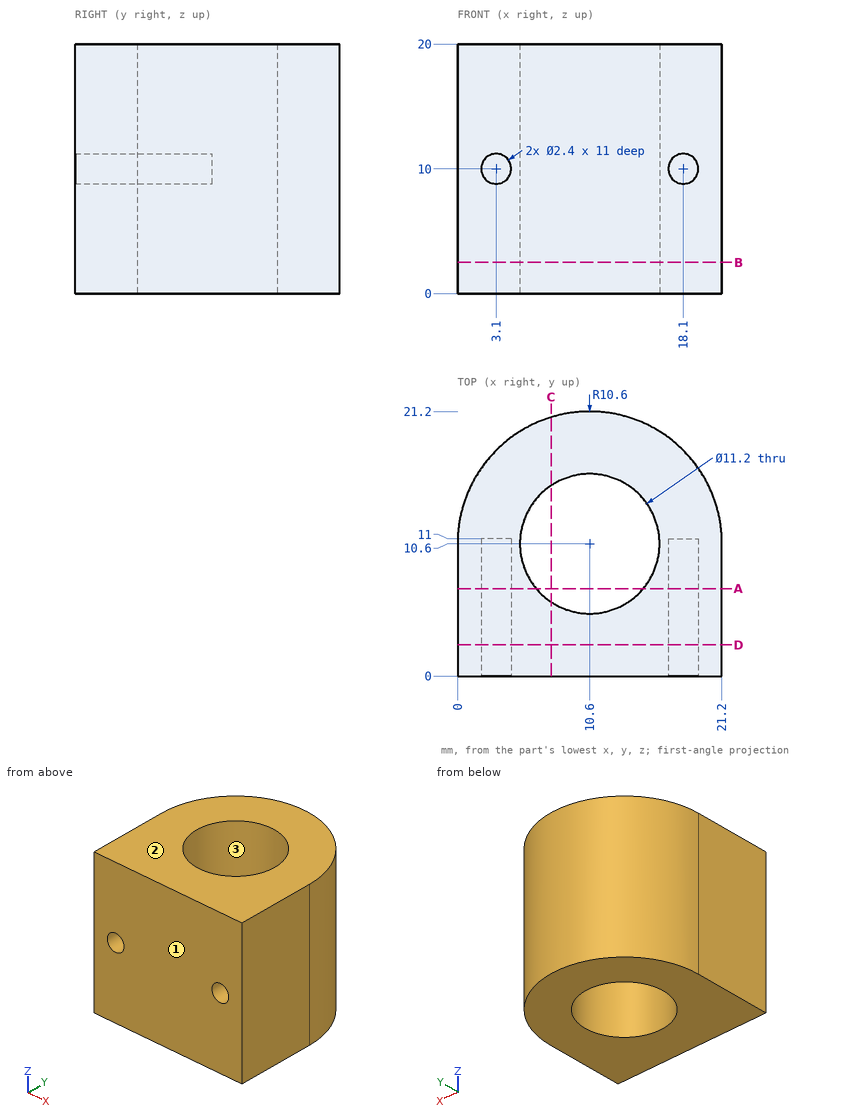
Study the drawing (mm; zero at the part's minimum x, y, z) and answer. Give positions to 0.01 mm unless a question says otherwise; leave off trailing zeros. Loops run counter-clockwise (first coordinate to the right, second up) from the corner with the lowest first, then second, coordinate; pieces in that order, holes last. Notation, with made-up numbers: M -4,3 L 26,3 A13 cw 26,27 Z; hole C 24,13 d2. An arc over 180 degrees is marked long. One line per item, written item: value.
1. Find the intervals of material crossed by probe 1 along X at (y, z) = (2.5, 10); probe 2 along X at (y, z) = (7.25, 10); probe 3 along X at (y, z) = (5.75, 10), in increasing order.
Found:
probe 1: 0 to 1.9, 4.3 to 16.9, 19.3 to 21.2
probe 2: 0 to 1.9, 4.3 to 6.11, 15.09 to 16.9, 19.3 to 21.2
probe 3: 0 to 1.9, 4.3 to 7.8, 13.4 to 16.9, 19.3 to 21.2
2. Section B-B on z = 2.5 is taken. Determine the outline of the cut face in (x, y).
Found:
outline: M 0,0 L 21.2,0 L 21.2,10.6 A10.6 ccw 0,10.6 Z; hole C 10.6,10.6 d11.2
3. Each of these flat-tipped pins is pushed along its axis until it touches: P1, Ø1.2, axis at x = 18.5, z = 10, coming from the -Y side; P2, Ø12, axis at x = 3, z = 12.5, coming from the +Y side; P3, Ø1.4, axis at x = 3.1, z = 10, coming from the +Y side. Where does it stop, or does it pass through?
Found:
P1: y = 11
P2: y = 21.08
P3: y = 18.73
4. For a pull along Y with two mould halves and no side action, classify the marked faces 1, 2 and 3 as pulls with the +Y half, pulls with the -Y half, needs draft (parallel to the pull), parting line crosses it, or undercut.
Found:
face 1: pulls with the -Y half
face 2: needs draft
face 3: undercut
5. Section A-A on y = 7 is taken. Determine the outline of the cut face in (x, z).
Found:
outline: M 0,0 L 6.31,0 L 6.31,20 L 0,20 Z; M 14.89,0 L 21.2,0 L 21.2,20 L 14.89,20 Z; hole C 3.1,10 d2.4; hole C 18.1,10 d2.4
6. Section D-D on y = 2.5 is taken. Determine the outline of the cut face in (x, z), plus the area to 3 significant figures.
Found:
outline: M 0,0 L 21.2,0 L 21.2,20 L 0,20 Z; hole C 3.1,10 d2.4; hole C 18.1,10 d2.4
area: 415 mm^2
7. Section C-C on x = 7.5 is taken. Determine the outline of the cut face in (y, z).
Found:
outline: M 0,0 L 5.94,0 L 5.94,20 L 0,20 Z; M 15.26,0 L 20.74,0 L 20.74,20 L 15.26,20 Z
